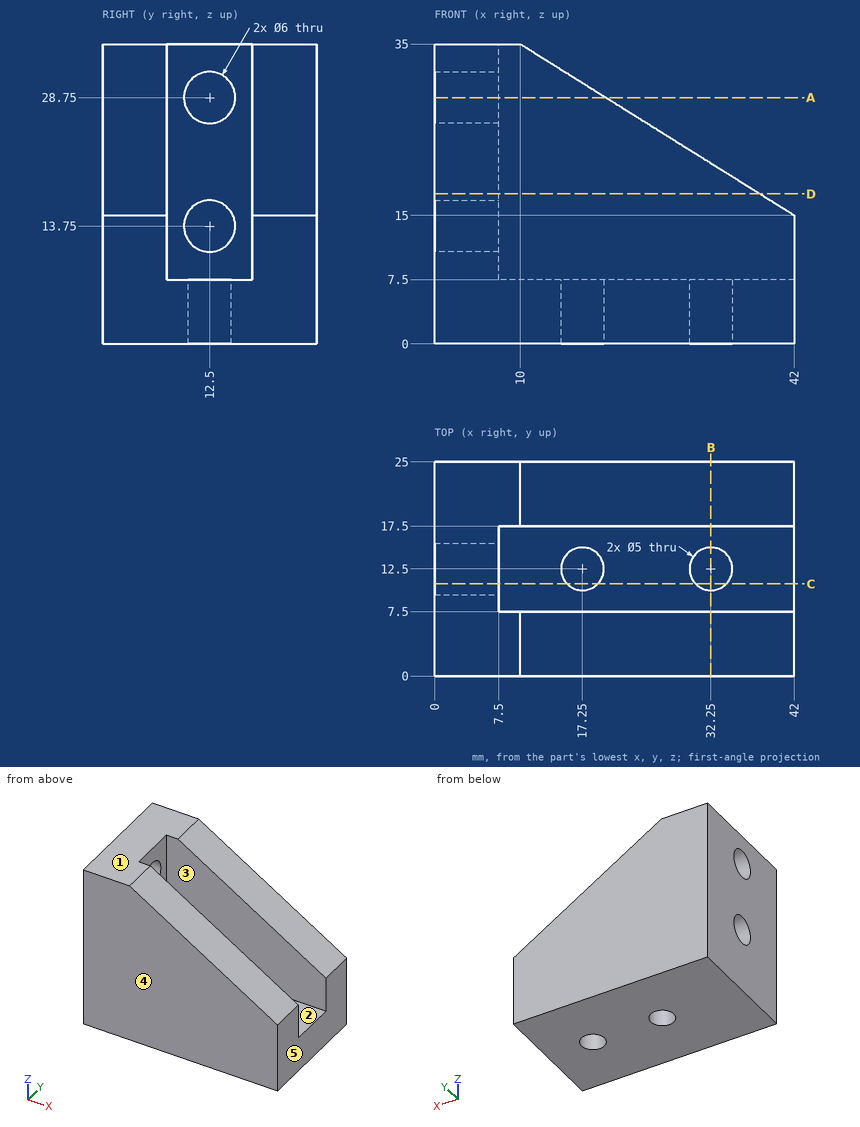
For this review, use the dimensioned drawing (mm, ordinates from the lowest corner) and the shaded views. A direction names the side the tool comes from. Round coordinates to 2 decimals unless told otherwise and drop trailing zeros. Write each loop counter-clockwise with the first axis right and the second up, starting at its lowest first coordinate (ties: lowest second). Pieces come first, ordered by that corner, then holes. Notation, with made-up numbers: M 47.5,26 L 54.5,26 A26 cw 54.5,58 Z; hole C 33,16.25 d8. An arc over 180 degrees is marked long. Answer as CSV lines item,"result". Start each with the question number.
Q1. Consider section C-C, the plane y = 10.75. Give the boundary of the cut face in (x, z), then the cut area to 3 significant figures.
Q2. Wall thickness on line 1 along Y through (x, z) = (3, 28.75); line 2 along Y through (x, z) = (27, 14); line 3 along Z through (x, y) = (11, 11): over which ranges is each line inside the solid? List them lowest first.
Q3. Clearance check with flat-ended pins moving along their axes: P1, Ø3.5, axis at y = 12.5, z = 13.75, coming from the +X side; P2, Ø5, axis at x = 18, y = 11, coming from the +Z side; P3, Ø5, axis at x = 36, y = 21.5, coming from the +Z side; P4, Ø5, axis at y = 11.5, z = 22, coming from the +X side. State where each tip first meets the part, or that it passes through.
Q4. Consider section A-A, the plane z = 28.75. Give the boundary of the cut face in (x, y).
Q5. Consider section D-D, the plane z = 17.5. Give the boundary of the cut face in (x, y), then the cut area to 3 significant figures.
Q6. Tool access review of the marked faces 1 and 2: name each direction out of +Z, -Z, +X, -X, +Y, -Y from which nothing blocks a thin tool from reaching the whole face with its end or side.
Q7. Consider section B-B, the plane x = 32.25. Give the boundary of the cut face in (y, z), then the cut area to 3 significant figures.
Q8. The part is to be moulded in two halves that separate along Y. For the marked faces 3, 4 and 5, say which applies: +Y half, -Y half, draft (parallel to the pull), parting line (faces both ways), or undercut.
Result set:
1,outline,"M 0,0 L 15.46,0 L 15.46,7.5 L 7.5,7.5 L 7.5,11.31 L 0,11.31 Z; M 0,16.19 L 7.5,16.19 L 7.5,26.31 L 0,26.31 Z; M 0,31.19 L 7.5,31.19 L 7.5,35 L 0,35 Z; M 19.04,0 L 30.46,0 L 30.46,7.5 L 19.04,7.5 Z; M 34.04,0 L 42,0 L 42,7.5 L 34.04,7.5 Z"
1,area,"395 mm²"
2,line 1,"y = 0 to 9.5, 15.5 to 25"
2,line 2,"y = 0 to 7.5, 17.5 to 25"
2,line 3,"z = 0 to 7.5"
3,P1,"passes through"
3,P2,"stops at z = 7.5"
3,P3,"stops at z = 20.31"
3,P4,"stops at x = 7.5"
4,outline,"M 0,0 L 20,0 L 20,7.5 L 7.5,7.5 L 7.5,9.5 L 0,9.5 Z; M 0,15.5 L 7.5,15.5 L 7.5,17.5 L 20,17.5 L 20,25 L 0,25 Z"
5,outline,"M 0,0 L 38,0 L 38,7.5 L 7.5,7.5 L 7.5,17.5 L 38,17.5 L 38,25 L 0,25 Z"
5,area,"645 mm²"
6,face 1,"+Z, +X, -X, +Y, -Y"
6,face 2,"+Z, +X"
7,outline,"M 0,0 L 10,0 L 10,7.5 L 7.5,7.5 L 7.5,21.09 L 0,21.09 Z; M 15,0 L 25,0 L 25,21.09 L 17.5,21.09 L 17.5,7.5 L 15,7.5 Z"
7,area,"354 mm²"
8,face 3,"undercut"
8,face 4,"-Y half"
8,face 5,"draft"
